Verification items for the finished model (mm, model axes). A direction names the side the tool comes from. Round coordinates to 2 decimals unless told otherwise and drop trailing zeros. Order: outer loops, then holes, each group sorted by start corner. A loop starts at its lowest first (then second) coordinate and runs counter-clockwise, first axis right, second up. Notation, with made-up numbers: M -18,15 L 10,15 A16 cw 10,38 Z; hole C 13,3.5 d6. An arc over 180 degrees is marked long. Write item = value, one per line. Start each with the question number.
from build123d import *

# Parameters (mm, degrees)
F0_W     = 80
F0_H     = 150
F0_W_2   = 130
F0_H_2   = 60
F1_DEPTH = 25
F2_W     = 240
F2_H     = 170
F3_DEPTH = 10
F4_W     = 20
F4_H     = 25
F5_DEPTH = 10
F6_R     = 2
F7_W     = 16
F7_H     = 21
F8_DEPTH = 10


with BuildPart() as f1:
    # F0 (on Top) → F1 (new body)
    with BuildSketch(Plane.XY):
        Polygon((105, -85), (120, -85), (120, 85), (-120, 85), (-120, -85), (25, -85), (25, -75), (20, -75), (20, -35), (110, -35), (110, -75), (105, -75), align=None)
        Polygon((110, 5), (110, -25), (10, -25), (10, -75), (-20, -75), (-20, -25), (-20, 5), align=None, mode=Mode.SUBTRACT)
        with Locations((-70, 0)):
            Rectangle(F0_W, F0_H, mode=Mode.SUBTRACT)
        with Locations((45, 45)):
            Rectangle(F0_W_2, F0_H_2, mode=Mode.SUBTRACT)
    extrude(amount=F1_DEPTH)

    # F2 (on face) → F3 (join)
    with BuildSketch(Plane(origin=(0, 0, 0), x_dir=(1, 0, 0), z_dir=(0, 0, -1))):
        Rectangle(F2_W, F2_H)
    extrude(amount=F3_DEPTH)

    # F4 (on face) → F5 (cut)
    with BuildSketch(Plane(origin=(0, -75, 0), x_dir=(-1, 0, 0), z_dir=(0, 1, 0))):
        with Locations((70, 12.5)):
            Rectangle(F4_W, F4_H)
    extrude(amount=-F5_DEPTH, mode=Mode.SUBTRACT)

    # F6
    f6_edges = [f1.edges().sort_by_distance(p)[0] for p in [
        (-110, 0, 25),
        (-120, 0, 25),
        (-100, -85, 25),
        (-95, -75, 25),
        (-60, -85, 12.5),
        (-80, -85, 12.5),
        (-80, -75, 12.5),
        (-60, -80, 25),
        (-60, -75, 12.5),
        (-30, 0, 25),
        (-45, -75, 25),
        (-70, -85, 0),
        (-20, -35, 25),
        (60, -25, 25),
        (-5, -75, 25),
        (10, -25, 12.5),
        (10, -50, 25),
        (25, -85, 12.5),
        (-17.5, -85, 25),
        (65, -85, 0),
        (105, -85, 12.5),
        (112.5, -85, 25),
        (120, 0, 25),
        (120, -85, 7.5),
        (-120, -85, 7.5),
        (45, 5, 25),
        (45, 15, 25),
        (-20, 45, 25),
        (-120, 85, 7.5),
        (120, 85, 7.5),
        (0, 85, 25),
        (45, 75, 25),
        (110, 45, 25),
        (110, -10, 25),
        (-80, -80, 25),
        (25, -80, 25),
        (105, -80, 25),
        (-70, 75, 25),
    ]]
    fillet(f6_edges, radius=F6_R)

    # F7 (on face) → F8 (cut)
    with BuildSketch(Plane.YZ.offset(20)):
        with Locations((-55, 14.5)):
            Rectangle(F7_W, F7_H)
    extrude(amount=-F8_DEPTH, mode=Mode.SUBTRACT)


solid = f1.part
1) Cross-section at A-A, the plane x = -45.5. Enter the section's corners in (y, z).
2) Cross-section at C-C, the plane y = 51. Enter the section's corners in (x, z).
3) Cross-section at D-D, the plane x = 34. Enter the section's corners in (y, z), then the cut area to 3 significant figures.
4) Release check for a two-part mould opening along Y. For faces 1 (the flat face through (-2, 85, 7)), 2 (the flat face through (-96, -75, 11)), 3 (the flat face through (-2, -1, -10)), 4 (the flat face through (30, -18, 0)) record: pulls with the +Y half, pulls with the -Y half, needs draft (parallel to the pull), parting line crosses it, or undercut.
5) Scan lines: probe 1 along X at (y, z) = (71.5, 15); probe 2 along Y at (x, z) = (-18, 21.5); probe 3 along X at (y, z) = (-33.5, 19). Record each from-to range of solid material in increasing order.
6) Cross-section at B-B, the plane y = -51.5. Enter the section's corners in (x, z).
7) Gauge pin test, flat ends, axial feed: P1, Ø7, axis at x = -74.5, z = 11, coming from the -Y side; P2, Ø11, axis at x = 15.5, y = -55, coming from the +Z side; P3, Ø6, axis at x = -1, y = -12.5, coming from the +Z side. Record the tip position at first contact, or that the pin passes through.
8) Access from +Z, -Z, +X, -X, +Y, -Y to the whole of each face (thin tool, end or side, straight path). Record for faces 5 (the flat face through (25, -79, 11)), 6 (the flat face through (23, -75, 12)).
Geometry results:
q1.outline = M -85,-10 L 85,-10 L 85,23 A2 ccw 83,25 L 77,25 A2 ccw 75,23 L 75,0 L -75,0 L -75,23 A2 ccw -77,25 L -83,25 A2 ccw -85,23 Z
q2.outline = M -120,-10 L 120,-10 L 120,23 A2 ccw 118,25 L 112,25 A2 ccw 110,23 L 110,0 L -20,0 L -20,23 A2 ccw -22,25 L -28,25 A2 ccw -30,23 L -30,0 L -110,0 L -110,23 A2 ccw -112,25 L -118,25 A2 ccw -120,23 Z
q3.outline = M -85,-10 L 85,-10 L 85,23 A2 ccw 83,25 L 77,25 A2 ccw 75,23 L 75,0 L 15,0 L 15,23 A2 ccw 13,25 L 7,25 A2 ccw 5,23 L 5,0 L -25,0 L -25,23 A2 ccw -27,25 L -35,25 L -35,0 L -83,0 A2 ccw -85,-2 Z
q3.area = 2,440 mm^2
q4.face_1 = pulls with the +Y half
q4.face_2 = undercut
q4.face_3 = needs draft
q4.face_4 = undercut
q5.probe_1 = -120 to -110, -30 to -20, 110 to 120
q5.probe_2 = -85 to -75, 5 to 15, 75 to 85
q5.probe_3 = -120 to -110, -30 to -20, 10 to 120
q6.outline = M -120,-10 L 120,-10 L 120,23 A2 ccw 118,25 L 110,25 L 110,0 L 20,0 L 20,4 L 10,4 L 10,0 L -20,0 L -20,23 A2 ccw -22,25 L -28,25 A2 ccw -30,23 L -30,0 L -110,0 L -110,23 A2 ccw -112,25 L -118,25 A2 ccw -120,23 Z
q7.P1 = 75
q7.P2 = 4
q7.P3 = 0
q8.face_5 = +Z, -Y
q8.face_6 = +Z
